Check sheet for the modelled part. Datum: model origin and axes. Units: mm. Face numbers are marked on the shaded views. A direction names the side the tool comes from. Round coordinates to 2 decimals unless told otherwise and drop trailing zeros. Write each loop counter-clockwise with the first axis right and the second up, starting at its lowest first coordinate (ties: lowest second). Pieces come first, ordered by that corner, then holes.
from build123d import *

# Parameters (mm, degrees)
BASE_FLANGE1_DEPTH = 2


# Sheet-metal steps are written as plain solids
with BuildPart() as part:
    # Sketch1 → Base-Flange1 (new, symmetric)
    with BuildSketch(Plane(origin=(0, 0, 0), x_dir=(0, 0, -1), z_dir=(1, 0, 0))):
        with BuildLine():
            Line((-3, 16), (-7.5, 16))
            ThreePointArc((-7.5, 16), (-7.853553391, 15.853553391), (-8, 15.5))
            Line((-8, 15.5), (-8, 4.5))
            ThreePointArc((-8, 4.5), (-7.853553391, 4.146446609), (-7.5, 4))
            Line((-7.5, 4), (-5.5, 4))
            ThreePointArc((-5.5, 4), (-4.792893219, 3.707106781), (-4.5, 3))
            Line((-4.5, 3), (-4.5, 2.207106781))
            ThreePointArc((-4.5, 2.207106781), (-4.461939766, 2.015765065), (-4.353553391, 1.853553391))
            Line((-4.353553391, 1.853553391), (-2.646446609, 0.146446609))
            ThreePointArc((-2.646446609, 0.146446609), (-2.484234935, 0.038060234), (-2.292893219, 0))
            Line((-2.292893219, 0), (2.292893219, 0))
            ThreePointArc((2.292893219, 0), (2.484234935, 0.038060234), (2.646446609, 0.146446609))
            Line((2.646446609, 0.146446609), (4.5, 2))
            Line((4.5, 2), (4.853553391, 1.646446609))
            Line((4.853553391, 1.646446609), (3, -0.207106781))
            ThreePointArc((3, -0.207106781), (2.675576651, -0.423879533), (2.292893219, -0.5))
            Line((2.292893219, -0.5), (-2.292893219, -0.5))
            ThreePointArc((-2.292893219, -0.5), (-2.675576651, -0.423879533), (-3, -0.207106781))
            Line((-3, -0.207106781), (-4.707106781, 1.5))
            ThreePointArc((-4.707106781, 1.5), (-4.923879533, 1.824423349), (-5, 2.207106781))
            Line((-5, 2.207106781), (-5, 3))
            ThreePointArc((-5, 3), (-5.146446609, 3.353553391), (-5.5, 3.5))
            Line((-5.5, 3.5), (-7.5, 3.5))
            ThreePointArc((-7.5, 3.5), (-8.207106781, 3.792893219), (-8.5, 4.5))
            Line((-8.5, 4.5), (-8.5, 15.5))
            ThreePointArc((-8.5, 15.5), (-8.207106781, 16.207106781), (-7.5, 16.5))
            Line((-7.5, 16.5), (-3, 16.5))
            Line((-3, 16.5), (-3, 16))
        make_face()
    extrude(amount=BASE_FLANGE1_DEPTH, both=True)


solid = part.part
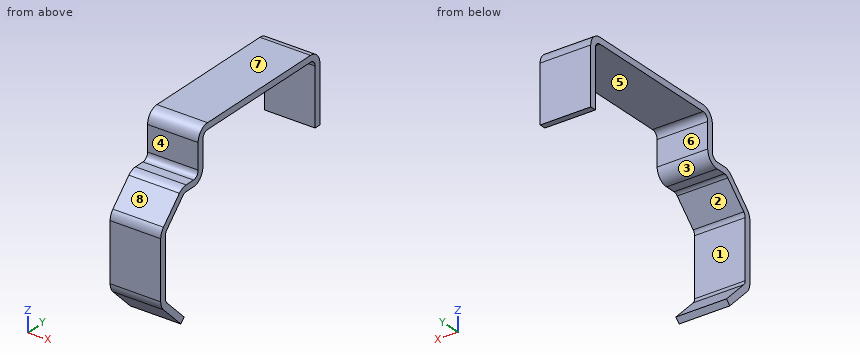
1. Set-up check for the marked faces 1, 2, 3 and 4: record each of +Z, -Z, +X, -X, +Y, -Y from which the full face is reachable in a straight line by a thin tool's end or side.
2. Sectioned sample at B-B, the plane y = 0.75. Enter the section's corners in (x, z), plus the area to 3 significant figures.
3. Go/stop test with flat-tipped pins: pin 1 (0.6 mm diameter, centred on x = 0.5, y = 16.5, fed in from -Z); pin 2 (2 mm diameter, centred on x = 0.5, z = -3.5, fed in from -Y); pin 3 (0.9 mm diameter, centred on x = 0.5, y = 2.5, fed in from +Z); pin 4 (8 mm diameter, centred on y = 8.5, z = 1, fed in from -X). Record where each tip stops, or that it passes through.
4. Sectioned sample at D-D, the plane z = 0.5. Enter the section's corners in (x, y), plus the area to 3 significant figures.
5. Scan lines: line 1 along Y through (x, z) = (-0.45, 7.5); line 2 along Z through (x, y) = (1.05, 10); line 3 along Z through (x, y) = (-1.1, 2.5). Record each from-to range of solid material in increasing order.
6. Sectioned sample at A-A, the plane z = 6.5. Enter the section's corners in (x, y).
7. Release check for a two-part mould opening along Y. For the marked faces 5, 6, 7 and 8 record: released by +Y, released by -Y, zero draft, split by the parting line, or undercut.
8. Sectioned sample at C-C, the plane x = -1.7. Enter the section's corners in (y, z).
Computed values:
1. face 1: +X, -X, +Y
1. face 2: +X, -X
1. face 3: -Z, +X, -X
1. face 4: +Z, +X, -X, -Y
2. outline: (-2, -3.96) - (2, -3.96) - (2, -3.25) - (-2, -3.25) - close; (-2, 3.25) - (2, 3.25) - (2, 3.96) - (-2, 3.96) - close
2. area: 5.66 mm2
3. pin 1: stops at z = 3
3. pin 2: stops at y = -0.48
3. pin 3: stops at z = 5
3. pin 4: passes through
4. outline: (-2, -0.5) - (2, -0.5) - (2, 0) - (-2, 0) - close
4. area: 2.00 mm2
5. line 1: y = 3.5 to 4, 16 to 16.5
5. line 2: z = 8 to 8.5
5. line 3: z = 4.5 to 5
6. outline: (-2, 3.5) - (2, 3.5) - (2, 4) - (-2, 4) - close; (-2, 16) - (2, 16) - (2, 16.5) - (-2, 16.5) - close
7. face 5: undercut
7. face 6: undercut
7. face 7: zero draft
7. face 8: released by -Y
8. outline: (-0.5, -2.29) arc R1 ccw to (-0.21, -3) - (1.65, -4.85) - (2, -4.5) - (0.15, -2.65) arc R0.5 cw to (0, -2.29) - (0, 2.29) arc R0.5 cw to (0.15, 2.65) - (1.85, 4.35) arc R0.5 cw to (2.21, 4.5) - (3, 4.5) arc R1 ccw to (4, 5.5) - (4, 7.5) arc R0.5 cw to (4.5, 8) - (15.5, 8) arc R0.5 cw to (16, 7.5) - (16, 3) - (16.5, 3) - (16.5, 7.5) arc R1 ccw to (15.5, 8.5) - (4.5, 8.5) arc R1 ccw to (3.5, 7.5) - (3.5, 5.5) arc R0.5 cw to (3, 5) - (2.21, 5) arc R1 ccw to (1.5, 4.71) - (-0.21, 3) arc R1 ccw to (-0.5, 2.29) - close
